Geometry: see drawing. Coordinates: mm, zero at the bounding-box minimum. A direction names the side the tool comes from. Round coordinates to 2 decimals unless told otherwise and drop trailing zeros. Write each loop counter-clockwise with the first axis right and the second up, starting at its lowest first coordinate (ties: lowest second). Pieces come first, ordered by that corner, then holes. Notation, with made-up numbers: M 88,88.5 L 122,88.5 A22 cw 122,103.5 Z; hole C -7,82.25 d11. An arc over 180 degrees is marked long. Use a Markdown table: item, result.
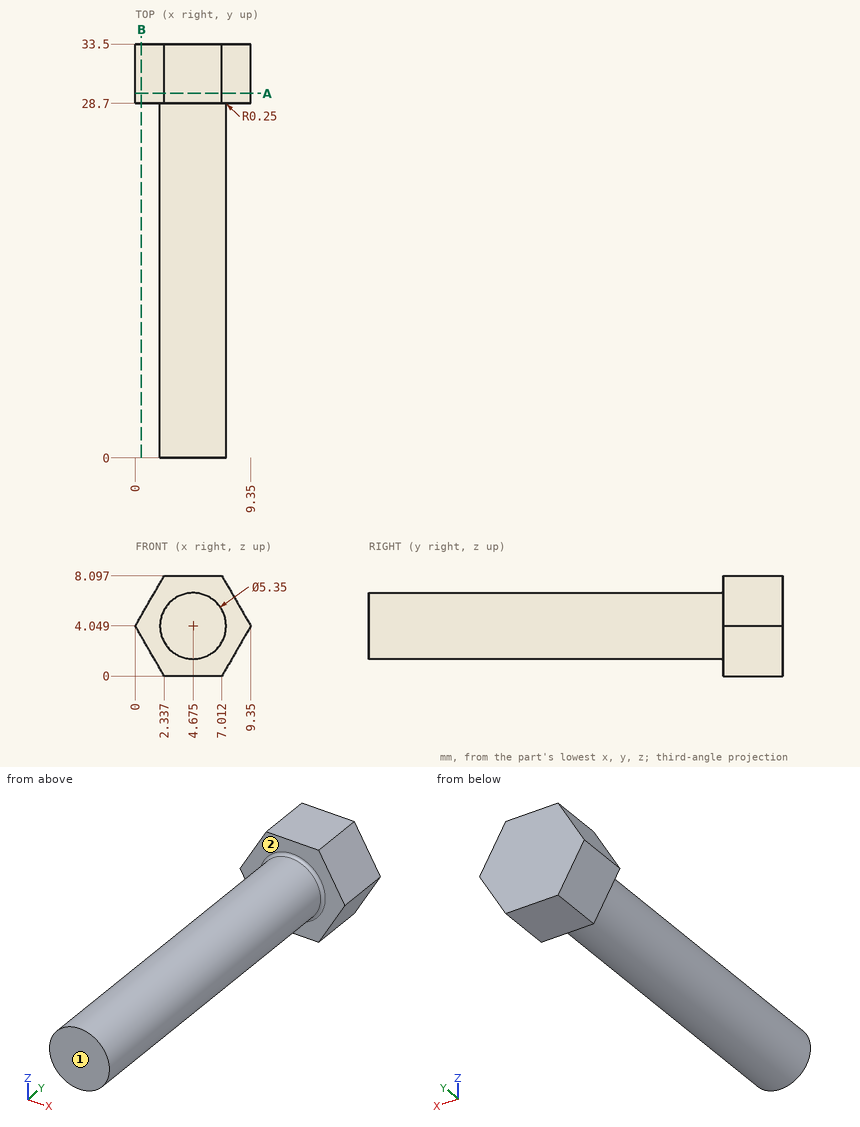
Q1. First-contact query: pin 1 Ø3 at (y, z) = (25.5, 7.5) entering from -X (1 decimal); pin 2 Ø1.5 at (x, y) = (4, 18) entering from +Z; pin 3 Ø3 at (y, z) = (10.5, 5.5) entering from -X. Flat tips, straight axial feed; report the tip coordinate or a pass-through.
Results are:
| item | result |
|---|---|
| pin 1 | x = 2.8 |
| pin 2 | z = 6.72 |
| pin 3 | x = 2 |
Q2. Reachability of the marked faces 1 and 2 from +Z, -Z, +X, -X, +Y, -Y: full face, straight path, thin tool, end or side. Return the list, or none.
Results are:
| item | result |
|---|---|
| face 1 | +Z, -Z, +X, -X, -Y |
| face 2 | -Y |
Q3. Section A-A on y = 29.5. Return loops of the section in (x, z).
Results are:
| item | result |
|---|---|
| outline | M 0,4.05 L 2.34,0 L 7.01,0 L 9.35,4.05 L 7.01,8.1 L 2.34,8.1 Z |
Q4. Section B-B on x = 0.5. Return loops of the section in (y, z) (1 decimal).
Results are:
| item | result |
|---|---|
| outline | M 28.7,3.2 L 33.5,3.2 L 33.5,4.9 L 28.7,4.9 Z |
Q5. Line query: L1, parallel to Y at x = 1.75, z = 6; L2, parallel to X at y = 31, z = 5.5; L3, parallel to X at y = 16, z = 3.25. Output: solid intervals per line, ascending.
Results are:
| item | result |
|---|---|
| L1 | 28.7 to 33.5 |
| L2 | 0.84 to 8.51 |
| L3 | 2.12 to 7.23 |
